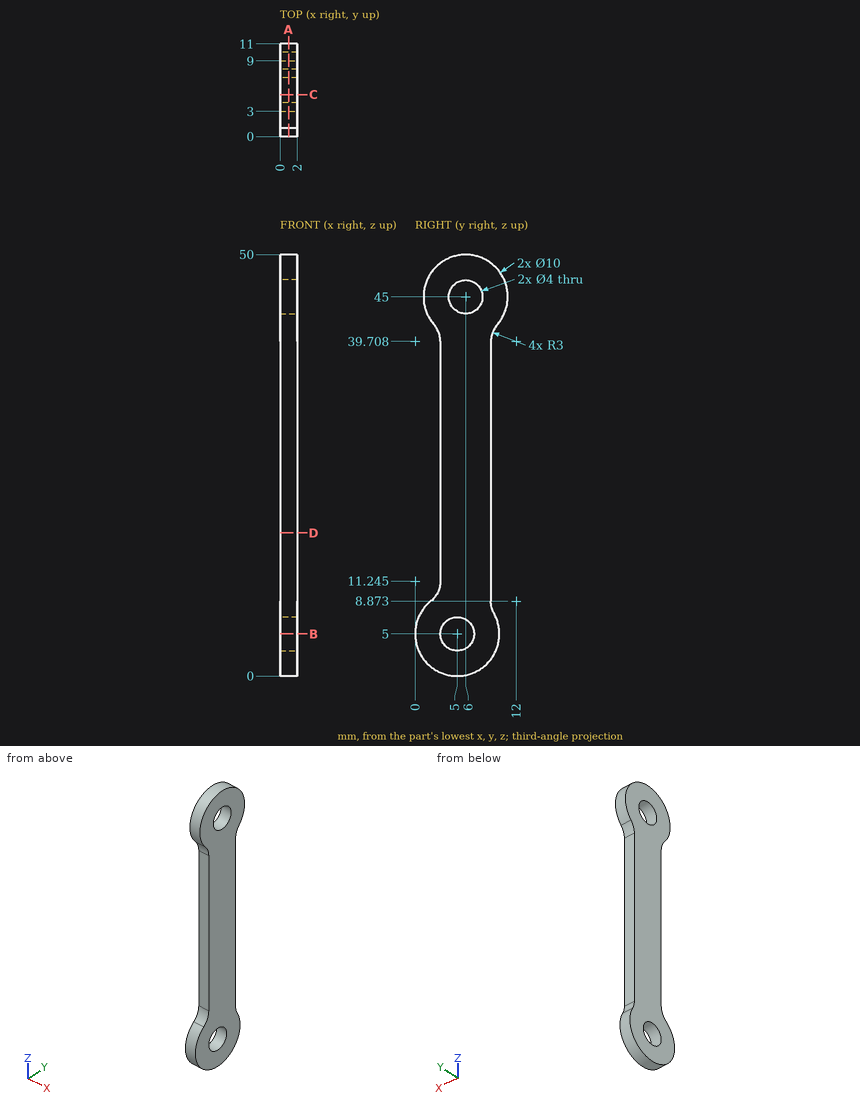
Geometry: see drawing. Coordinates: mm, zero at the bounding-box minimum. Give positions to 0.01 mm unless a question says otherwise; leave off trailing zeros. Write each loop counter-clockwise with the first axis right and the second up, starting at its lowest first coordinate (ties: lowest second). Pieces come first, ordered by that corner, then holes. Notation, with made-up numbers: (38.5, -7) -> (62.5, -7) arc R29 cw to (62.5, 16) -> close; hole circle Ø3 at (16.5, 21). An arc over 180 degrees is marked (long way). Use one line per item in the form item = value. Start each with the question number.
1) Ray query, probe 1 along Z at (x, y) = (0.6, 6); probe 2 along Z at (x, y) = (1.15, 6.5) (1 decimal); probe 3 along Y at (x, z) = (1, 45). Return the intervals inside material, ascending. Write a range as from..to.
2) Pin query (flat end, axial travel): pin 1 (1 mm diameter, centred on x = 1, z = 20, fed in from +Y). Return the tip coordinate at first contact, or that it passes through.
3) Section query A-A on x = 1. Count the separate pieces of the cut face and the enclosed holes in it.
4) Section query C-C on y = 5. Return the cut outline in (x, z).
5) Section query B-B on z = 5. Return the cut outline in (x, y), then the cut area to 3 significant figures.
6) Section query D-D on z = 17. Return the cut outline in (x, y).
Outcome:
q1.probe_1 = 0.1..3.27, 6.73..43, 47..50
q1.probe_2 = 0.2..3.7, 6.3..43.1, 46.9..50
q1.probe_3 = 1..4, 8..11
q2.pin_1 = 9
q3.separate_pieces = 1
q3.enclosed_holes = 2
q4.outline = (0, 0) -> (2, 0) -> (2, 3) -> (0, 3) -> close; (0, 7) -> (2, 7) -> (2, 43.27) -> (0, 43.27) -> close; (0, 46.73) -> (2, 46.73) -> (2, 49.9) -> (0, 49.9) -> close
q5.outline = (0, 0) -> (2, 0) -> (2, 3) -> (0, 3) -> close; (0, 7) -> (2, 7) -> (2, 10) -> (0, 10) -> close
q5.area = 12.0 mm^2
q6.outline = (0, 3) -> (2, 3) -> (2, 9) -> (0, 9) -> close
